from build123d import *

# Parameters (mm, degrees)
SKETCH_1_R          = 25
SKETCH_1_R_2        = 22.5
EXTRUDE_1_DEPTH     = 250
SKETCH_2_R          = 24
CUT_EXTRUDE_1_DEPTH = 22
CUT_EXTRUDE_START   = -22
SKETCH_3_R          = 24
CUT_EXTRUDE_2_DEPTH = 22
SKETCH_4_R          = 24
SKETCH_4_R_2        = 23.95
EXTRUDE_2_DEPTH     = 22


with BuildPart() as part:
    # Эскиз1 → Бобышка-Вытянуть1 (new body)
    with BuildSketch(Plane(origin=(0, 0, 0), x_dir=(1, 0, 0), z_dir=(0, 1, 0))):
        with Locations(Location((0, 0, 0), (0, 0, 270))):
            Circle(SKETCH_1_R)
        with Locations(Location((0, 0, 0), (0, 0, 270))):
            Circle(SKETCH_1_R_2, mode=Mode.SUBTRACT)
    extrude(amount=EXTRUDE_1_DEPTH)

    # Эскиз2 → Вырез-Вытянуть1 (cut)
    with BuildSketch(Plane.XZ):
        with Locations(Location((0, 0, 0), (0, 0, 270))):
            Circle(SKETCH_2_R)
    extrude(amount=-CUT_EXTRUDE_1_DEPTH, mode=Mode.SUBTRACT)

    # Эскиз3 → Вырез-Вытянуть2 (cut)
    with BuildSketch(Plane(origin=(0, 250, 0), x_dir=(1, 0, 0), z_dir=(0, 1, 0)).offset(CUT_EXTRUDE_START)):
        with Locations(Location((0, 0, 0), (0, 0, 90))):
            Circle(SKETCH_3_R)
    extrude(amount=CUT_EXTRUDE_2_DEPTH, mode=Mode.SUBTRACT)

    # Эскиз4 → Бобышка-Вытянуть2 (add)
    with BuildSketch(Plane(origin=(0, 228, 0), x_dir=(1, 0, 0), z_dir=(0, 1, 0))):
        with Locations(Location((0, 0, 0), (0, 0, 90))):
            Circle(SKETCH_4_R)
        with Locations(Location((0, 0, 0), (0, 0, 270))):
            Circle(SKETCH_4_R_2, mode=Mode.SUBTRACT)
    extrude(amount=EXTRUDE_2_DEPTH)


solid = part.part
Input: part model. Units: mm. Frame: model coordinates. A direction names the side the tool comes from. Coordinates: 2 decimals unless noted, no trailing zeros. Order: outer loops, then holes, each group sorted by start corner. A loop starts at its lowest first (then second) coordinate and runs counter-clockwise, first axis right, second up. Notation, with made-up numbers: M -24.75,16 L -14.75,16 A3 cw -14.75,20 Z; hole C 83,-40 d9. An arc over 180 degrees is marked long. Answer as CSV lines item,"result".
1. First-contact query: P1, Ø8, axis at y = 36.5, z = 18, coming from the -X side; P2, Ø8, axis at y = 211, z = 6.5, coming from the -X side; P3, Ø6, axis at y = 205.5, z = -3, coming from the -X side. Flat tips, straight axial feed; report the tip coordinate or a pass-through.
Reported:
P1,"x = -20.71"
P2,"x = -24.87"
P3,"x = -25"
2. Section C-C (y = 70.5). Return the cut outline in (x, z), then the cut area to 3 significant figures.
Reported:
outline,"C 0,0 d50; hole C 0,0 d45"
area,"373 mm2"
3. Material intervals for line 1 (X direction, y = 96.5, z = 0); line 2 (Z direction, x = 1.5, y = 83.5); line 3 (X direction, y = 8, z = 0), sorted ascending. Write a range as from..to.
Reported:
line 1,"-25..-22.5, 22.5..25"
line 2,"-24.95..-22.45, 22.45..24.95"
line 3,"-25..-24, 24..25"
4. Section A-A (z = 0). Return the cut outline in (x, y), then the cut area to 3 significant figures.
Reported:
outline,"M -25,0 L -24,0 L -24,22 L -22.5,22 L -22.5,228 L -23.95,228 L -23.95,250 L -25,250 Z; M 22.5,22 L 24,22 L 24,0 L 25,0 L 25,250 L 23.95,250 L 23.95,228 L 22.5,228 Z"
area,"1,120 mm2"
5. Access query for faces 4 (the cylindrical face through (-8.618, 123.558, 20.784)), 5 (the cylindrical face through (-23.38, 238.85, -5.19)), 6 (the cylindrical face through (7.21, 10.85, -22.89)). Directions: +Z, -Z, +X, -X, +Y, -Y. A direction counts if a zero-diameter tool reaches every point of the face in a straight line with its end or side. Return the directions, or none.
Reported:
face 4,"+Y, -Y"
face 5,"+Y"
face 6,"-Y"
6. Pull-direction query (Z, two-part tool) for faces 1 (the flat face through (9.4, 0, -22.3)), 2 (the flat face through (-18, 22, -14)), 3 (the cylindrical face through (7.509, 123.25, 23.846)); classes: released by +Z, released by -Z, zero draft, split by the parting line, or undercut.
Reported:
face 1,"zero draft"
face 2,"undercut"
face 3,"split by the parting line"
7. Section B-B (x = 0). Return the cut outline in (y, z).
Reported:
outline,"M 0,-25 L 250,-25 L 250,-23.95 L 228,-23.95 L 228,-22.5 L 22,-22.5 L 22,-24 L 0,-24 Z; M 0,24 L 22,24 L 22,22.5 L 228,22.5 L 228,23.95 L 250,23.95 L 250,25 L 0,25 Z"
